For this review, take the finished solid that the model builds, in its own axes (mm). Round coordinates to 2 decimals unless told otherwise and drop trailing zeros. Order: outer loops, then holes, each group sorted by start corner. A loop starts at its lowest first (then second) coordinate and runs counter-clockwise, first axis right, second up. Notation, with made-up numbers: M 55.25,30.5 L 70.25,30.5 A19 cw 70.25,51.5 Z; hole C 30.25,-27.5 d5. An arc over 180 degrees is marked long. Answer as a JSON object with one key per item and string values.
from build123d import *

# Parameters (mm, degrees)
ESQUISSE1_W                     = 57.15
ESQUISSE1_H                     = 127
BOSS_EXTRU_1_DEPTH              = 6.35
ESQUISSE2_W                     = 6.35
ESQUISSE2_H                     = 12.7
BOSS_EXTRU_2_DEPTH              = 6.35
R_P_TITION_LIN_AIRE1_COUNT      = 4
R_P_TITION_LIN_AIRE1_PITCH      = 25.4
ESQUISSE3_W                     = 12.7
ESQUISSE3_H                     = 6.35
ENL_V_MAT_EXTRU_1_DEPTH         = 6.35
R_P_TITION_LIN_AIRE2_COUNT      = 2
R_P_TITION_LIN_AIRE2_PITCH      = 25.4
R_P_TITION_LIN_AIRE2_COUNT_DIR2 = 2
R_P_TITION_LIN_AIRE2_PITCH_DIR2 = 57.15


with BuildPart() as part:
    # Esquisse1 → Boss.-Extru.1 (new body)
    with BuildSketch(Plane.XY):
        Rectangle(ESQUISSE1_W, ESQUISSE1_H)
    extrude(amount=BOSS_EXTRU_1_DEPTH)

    # Esquisse2 → Boss.-Extru.2 (add)
    with BuildSketch(Plane.XY.offset(6.35)):
        with Locations((31.75, 44.45)):
            Rectangle(ESQUISSE2_W, ESQUISSE2_H)
    boss_extru_2 = extrude(amount=-BOSS_EXTRU_2_DEPTH)

    # Répétition linéaire1: Boss.-Extru.2 ×4
    with Locations(*[(0, -i * R_P_TITION_LIN_AIRE1_PITCH, 0) for i in range(1, R_P_TITION_LIN_AIRE1_COUNT)]):
        add(boss_extru_2)

    # Esquisse3 → Enlèv. mat.-Extru.1 (cut)
    with BuildSketch(Plane.XY.offset(6.35)):
        with Locations((-12.7, 9.525)):
            Rectangle(ESQUISSE3_W, ESQUISSE3_H)
    enl_v_mat_extru_1 = extrude(amount=-ENL_V_MAT_EXTRU_1_DEPTH, mode=Mode.SUBTRACT)

    # Répétition linéaire2: Enl_v. mat.-Extru.1 2 × 2
    with Locations(*[(i * R_P_TITION_LIN_AIRE2_PITCH, j * R_P_TITION_LIN_AIRE2_PITCH_DIR2, 0) for i in range(R_P_TITION_LIN_AIRE2_COUNT) for j in range(R_P_TITION_LIN_AIRE2_COUNT_DIR2) if (i, j) != (0, 0)]):
        add(enl_v_mat_extru_1, mode=Mode.SUBTRACT)


solid = part.part
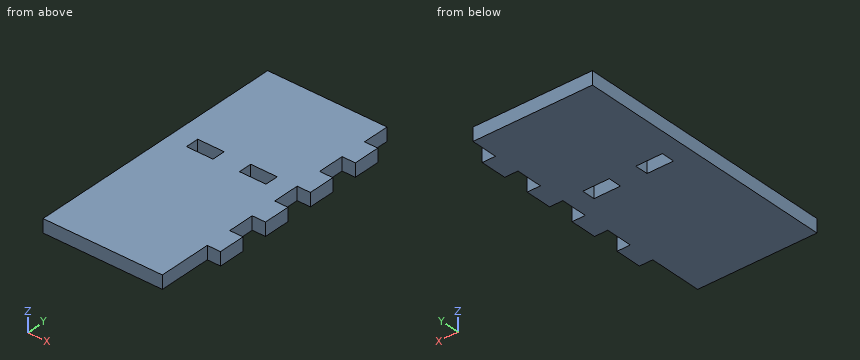
1) Add section B-B on x = 30. State the section outline as (y, z) points, and give its area (3 significant figures).
Geometry check:
{"outline": "M -38.1,0 L -25.4,0 L -25.4,6.35 L -38.1,6.35 Z; M -12.7,0 L 0,0 L 0,6.35 L -12.7,6.35 Z; M 12.7,0 L 25.4,0 L 25.4,6.35 L 12.7,6.35 Z; M 38.1,0 L 50.8,0 L 50.8,6.35 L 38.1,6.35 Z", "area": "323 mm²"}
2) Add section D-D on z = 3.5. State the section outline as (x, y) points (3 decimals).
Geometry check:
{"outline": "M -28.575,-63.5 L 28.575,-63.5 L 28.575,-38.1 L 34.925,-38.1 L 34.925,-25.4 L 28.575,-25.4 L 28.575,-12.7 L 34.925,-12.7 L 34.925,0 L 28.575,0 L 28.575,12.7 L 34.925,12.7 L 34.925,25.4 L 28.575,25.4 L 28.575,38.1 L 34.925,38.1 L 34.925,50.8 L 28.575,50.8 L 28.575,63.5 L -28.575,63.5 Z; hole M -19.05,6.35 L -6.35,6.35 L -6.35,12.7 L -19.05,12.7 Z; hole M 6.35,6.35 L 19.05,6.35 L 19.05,12.7 L 6.35,12.7 Z"}
3) Insertion check: P1, Ø3, axis at y = 10.5, z = 2.5, coming from the +X side (3 decimals); P2, Ø1.9, axis at x = 32, z = 4.5, coming from the +Y side; P3, Ø3, axis at x = 31.5, z = 3.5, coming from the -Y side. Each pin has a flat end and moves straight along its axis. Give the tip position at first contact, or say it passes through.
Geometry check:
{"P1": "stops at x = 28.575", "P2": "stops at y = 50.8", "P3": "stops at y = -38.1"}
4) Add section C-C on x = -10. State the section outline as (y, z) points, and give its area (3 significant figures).
Geometry check:
{"outline": "M -63.5,0 L 6.35,0 L 6.35,6.35 L -63.5,6.35 Z; M 12.7,0 L 63.5,0 L 63.5,6.35 L 12.7,6.35 Z", "area": "766 mm²"}
5) For L1, parallel to Y at x = 30, z = 2.75; L2, parallel to Y at x = 10, z = 5.5; L3, parallel to X at y = 55.5, z = 4.25 (3 decimals), list the stretches that pass through material, from the lowest coordinate up.
Geometry check:
{"L1": "y = -38.1 to -25.4, -12.7 to 0, 12.7 to 25.4, 38.1 to 50.8", "L2": "y = -63.5 to 6.35, 12.7 to 63.5", "L3": "x = -28.575 to 28.575"}
6) Add section A-A on y = 8.5. State the section outline as (x, z) points (3 decimals), and give its area (3 significant figures).
Geometry check:
{"outline": "M -28.575,0 L -19.05,0 L -19.05,6.35 L -28.575,6.35 Z; M -6.35,0 L 6.35,0 L 6.35,6.35 L -6.35,6.35 Z; M 19.05,0 L 28.575,0 L 28.575,6.35 L 19.05,6.35 Z", "area": "202 mm²"}
